Check sheet for the modelled part. Datum: model origin and axes. Units: mm. A direction names the side the tool comes from. Give positions to 0.01 mm unless a question says otherwise; leave off trailing zeros. Order: outer loops, then holes, each group sorted by start corner. A loop starts at its lowest first (then second) coordinate and runs counter-clockwise, first axis right, second up. Notation, with made-up numbers: (79.25, 63) -> (136.25, 63) arc R5 cw to (136.25, 69) -> close; hole circle Ø1 at (89.25, -37.5). An arc over 180 degrees is marked (long way). Write each question's results on one line, items separated by ' | '.
from build123d import *

# Parameters (mm, degrees)
F0_W      = 152.4
F0_H      = 152.4
F1_DEPTH  = 38.1
F2_W      = 76.2
F2_H      = 76.2
F3_DEPTH  = 38.1
F4_W      = 38.1
F4_H      = 38.1
F5_DEPTH  = 1143
F6_W      = 152.4
F6_H      = 152.4
F7_DEPTH  = 38.1
F8_R      = 6.35
F9_DEPTH  = 0.254
F10_R     = 19.05
F11_DEPTH = 0.254


with BuildPart() as f1:
    # F0 (on Top) → F1 (new body)
    with BuildSketch(Plane.XY):
        Rectangle(F0_W, F0_H)
    extrude(amount=-F1_DEPTH)

    # F2 (on face) → F3 (cut)
    with BuildSketch(Plane.XY):
        Rectangle(F2_W, F2_H)
    extrude(amount=-F3_DEPTH, mode=Mode.SUBTRACT)

    # F4 (on face) → F5 (join)
    with BuildSketch(Plane.XY):
        with Locations((-57.15, -57.15)):
            Rectangle(F4_W, F4_H)
        with Locations((-57.15, 57.15)):
            Rectangle(F4_W, F4_H)
        with Locations((57.15, 57.15)):
            Rectangle(F4_W, F4_H)
        with Locations((57.15, -57.15)):
            Rectangle(F4_W, F4_H)
    extrude(amount=F5_DEPTH)

    # F6 (on face) → F7 (join)
    with BuildSketch(Plane.XY.offset(1143)):
        Rectangle(F6_W, F6_H)
    extrude(amount=F7_DEPTH)

    # F8 (on face) → F9 (join)
    with BuildSketch(Plane(origin=(-76.2, 0, 0), x_dir=(0, -1, 0), z_dir=(-1, 0, 0))):
        with Locations((-57.15, -19.05)):
            Circle(F8_R)
        with Locations((57.15, -19.05)):
            Circle(F8_R)
    extrude(amount=F9_DEPTH)

    # F10 (on face) → F11 (cut)
    with BuildSketch(Plane.XY.offset(1181.1)):
        Circle(F10_R)
    extrude(amount=-F11_DEPTH, mode=Mode.SUBTRACT)


solid = f1.part
1. Section check A-A on z = 977.5. Record the cut outline in (x, y).
Verdict:
outline: (-76.2, -76.2) -> (-38.1, -76.2) -> (-38.1, -38.1) -> (-76.2, -38.1) -> close; (-76.2, 38.1) -> (-38.1, 38.1) -> (-38.1, 76.2) -> (-76.2, 76.2) -> close; (38.1, -76.2) -> (76.2, -76.2) -> (76.2, -38.1) -> (38.1, -38.1) -> close; (38.1, 38.1) -> (76.2, 38.1) -> (76.2, 76.2) -> (38.1, 76.2) -> close
2. Material ranges on probe 1 along Z at (x, y) = (-56, -11); probe 2 along X at (y, z) = (-51.5, 201); probe 3 along Y at (x, z) = (0, 1181), recorded low to high. Write a range as from..to.
Verdict:
probe 1: z = -38.1..0, 1143..1181.1 | probe 2: x = -76.2..-38.1, 38.1..76.2 | probe 3: y = -76.2..-19.05, 19.05..76.2
3. Mould release check, pull along X, two halves, no side actions. Record for faces 1 (the flat face through (38.1, -57, 563)), 2 (the flat face through (57, 38.1, 563)), 3 (the flat face through (76.2, -52, 563)), 4 (the flat face through (-38.1, 57, 563)): +X half, -X half, draft (parallel to the pull), parting line (faces both ways), or undercut.
Verdict:
face 1: undercut | face 2: draft | face 3: +X half | face 4: undercut
4. Section check D-D on x = 58. Record the cut outline in (y, z), then the cut area to 3 significant figures.
Verdict:
outline: (-76.2, -38.1) -> (76.2, -38.1) -> (76.2, 1181.1) -> (-76.2, 1181.1) -> close; hole (-38.1, 0) -> (38.1, 0) -> (38.1, 1143) -> (-38.1, 1143) -> close | area: 98,700 mm^2
5. Gauge pin test, flat ends, axial feed: pin 1 Ø10 at (y, z) = (-32, 241.5) entering from -X; pin 2 Ø11.5 at (x, y) = (-5, -7.5) entering from +Z; pin 3 Ø12 at (y, z) = (-34, 519) entering from -X. Record the tip position at first contact, or that the pin passes through.
Verdict:
pin 1: passes through | pin 2: stops at z = 1180.85 | pin 3: stops at x = -76.2
6. Section check B-B on y = 0. Record the cut outline in (x, z), then the cut area to 3 significant figures.
Verdict:
outline: (-76.2, -38.1) -> (-38.1, -38.1) -> (-38.1, 0) -> (-76.2, 0) -> close; (-76.2, 1143) -> (76.2, 1143) -> (76.2, 1181.1) -> (19.05, 1181.1) -> (19.05, 1180.85) -> (-19.05, 1180.85) -> (-19.05, 1181.1) -> (-76.2, 1181.1) -> close; (38.1, -38.1) -> (76.2, -38.1) -> (76.2, 0) -> (38.1, 0) -> close | area: 8,700 mm^2
7. Access from +Z, -Z, +X, -X, +Y, -Y to the whole of each face (thin tool, end or side, straight path). Record for faces 5 (the flat face through (-1, 38.1, -19)), 6 (the flat face through (-57, 1, 0)), 7 (the flat face through (-52, -76.2, 563)), 8 (the flat face through (-38.1, -57, 563)).
Verdict:
face 5: -Z | face 6: +X, -X | face 7: +Z, -Z, +X, -X, -Y | face 8: +Y, -Y
